Geometry: final body of the model. Coordinates: model frame, mm. Face numbers are marked on the shaded views. Coordinates: 2 decimals unless noted, no trailing zeros. Order: outer loops, then holes, each group sorted by start corner. A loop starts at its lowest first (then second) coordinate and runs counter-clockwise, first axis right, second up. Notation, with made-up numbers: M -37,40.25 L -1,40.25 A28 cw -1,61.25 Z; hole C 73,3 d8. An arc over 180 degrees is marked long. Use CSV: the item, a comma, the result in double quotes. Start each with the question number.
Q1. Ray query, probe 1 along X at (y, z) = (3.5, 0.25); probe 2 along Y at (x, z) = (2, -3.5); probe 3 along X at (y, z) = (3, -6.5). Return the intervals inside material, ascending.
Q2. Section query A-A, the plane y = 2.5. Output: boundary loops of the cut face in (x, z), and give its area (3 significant figures).
Q3. Section query B-B, the plane z = -0.25. Output: boundary loops of the cut face in (x, y), and give its area (4 significant figures).
Q4. First-contact query: P1, Ø8, axis at x = 2.5, z = -2, coming from the +Y side. Flat tip, straight axial feed; report the tip coordinate or a pass-through.
Q5. Mould query, pull axis X, two halves, no side actions, for the marked faces 1, 2, 3 and 4. Classes: +X half, -X half, draft (parallel to the pull), parting line (faces both ways), or undercut.
Q6. Section query D-D, the plane x = 8. Output: boundary loops of the cut face in (y, z).
Q7. Section query C-C, the plane y = 0. Output: boundary loops of the cut face in (x, z).
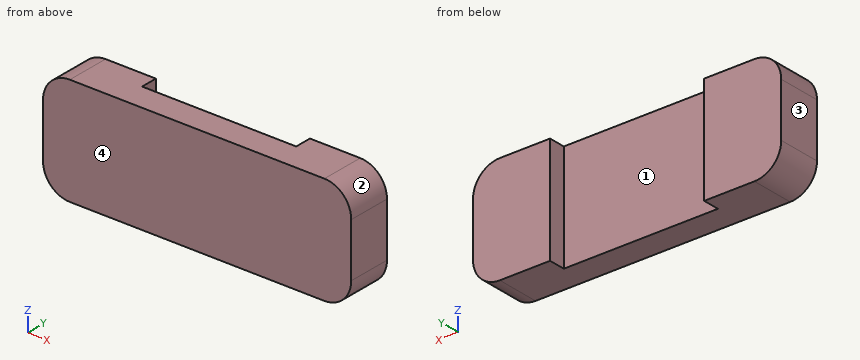
from build123d import *

# Parameters (mm, degrees)
SALIENTE_EXTRUIR1_DEPTH      = 4.5
SALIENTE_EXTRUIR1_DEPTH_BACK = 2
CROQUIS2_W                   = 23
CROQUIS2_H                   = 20.20150629
CORTAR_EXTRUIR1_DEPTH        = 2.5


with BuildPart() as part:
    # Croquis1 → Saliente-Extruir1 (new, two sides: drawn at the far end of the back side and taken through both)
    with BuildSketch(Plane(origin=(0, 0, 0), x_dir=(1, 0, 0), z_dir=(0, 1, 0)).offset(-SALIENTE_EXTRUIR1_DEPTH_BACK)):
        with BuildLine():
            Line((-19, 8), (19, 8))
            ThreePointArc((19, 8), (21.828427125, 6.828427125), (23, 4))
            Line((23, 4), (23, -4))
            ThreePointArc((23, -4), (21.828427125, -6.828427125), (19, -8))
            Line((19, -8), (-19, -8))
            ThreePointArc((-19, -8), (-21.828427125, -6.828427125), (-23, -4))
            Line((-23, -4), (-23, 4))
            ThreePointArc((-23, 4), (-21.828427125, 6.828427125), (-19, 8))
        make_face()
    extrude(amount=SALIENTE_EXTRUIR1_DEPTH + SALIENTE_EXTRUIR1_DEPTH_BACK)

    # Croquis2 → Cortar-Extruir1 (cut)
    with BuildSketch(Plane(origin=(0, 4.5, 0), x_dir=(1, 0, 0), z_dir=(0, 1, 0))):
        Rectangle(CROQUIS2_W, CROQUIS2_H)
    extrude(amount=-CORTAR_EXTRUIR1_DEPTH, mode=Mode.SUBTRACT)


solid = part.part
Responses:
1,probe 1,"x = -23 to -11.5, 11.5 to 23"
1,probe 2,"y = -2 to 2"
1,probe 3,"x = -22.12 to -11.5, 11.5 to 22.12"
2,outline,"M -23,-4 A4 ccw -19,-8 L -11.5,-8 L -11.5,8 L -19,8 A4 ccw -23,4 Z; M 11.5,-8 L 19,-8 A4 ccw 23,-4 L 23,4 A4 ccw 19,8 L 11.5,8 Z"
2,area,"354 mm²"
3,outline,"M -23,-2 L 23,-2 L 23,4.5 L 11.5,4.5 L 11.5,2 L -11.5,2 L -11.5,4.5 L -23,4.5 Z"
3,area,"241.5 mm²"
4,P1,"stops at y = 2"
5,face 1,"undercut"
5,face 2,"+X half"
5,face 3,"-X half"
5,face 4,"draft"
6,outline,"M -2,-8 L 2,-8 L 2,8 L -2,8 Z"
7,outline,"M -23,-4 A4 ccw -19,-8 L 19,-8 A4 ccw 23,-4 L 23,4 A4 ccw 19,8 L -19,8 A4 ccw -23,4 Z"
